Geometry check sheet. Reference: the model listing, model coordinates, mm. A direction names the side the tool comes from. Round coordinates to 2 decimals unless told otherwise and drop trailing zeros. Loops run counter-clockwise (first coordinate to the right, second up) from the corner with the lowest first, then second, coordinate; pieces in that order, holes last.
Autodesk Inventor part; units mm, degrees
ref_plane "YZ Plane" through (0, 0, 0) normal (1, 0, 0) x (0, 1, 0)
ref_plane "XZ Plane" through (0, 0, 0) normal (0, 1, 0) x (-1, 0, 0)
ref_plane "XY Plane" through (0, 0, 0) normal (0, 0, 1) x (1, 0, 0)
sketch "Sketch1" plane through (0, 0, 0) normal (0, 1, 0) x (-1, 0, 0)
  circle A0 centre (0, 0) radius 2.6
  line L0 (0, 0) -> (0, -2.6) construction
  line L1 (0, 0) -> (-2.6, 0) construction
  circle A1 centre (-20, 0) radius 2.6
  circle A2 centre (0, 40) radius 2.6
  circle A3 centre (-20, 40) radius 2.6
  circle A4 centre (0, 80) radius 2.6
  circle A5 centre (-20, 80) radius 2.6
  circle A6 centre (0, -25) radius 2.6
  line L2 (0, -25) -> (2.6, -25) construction
  line L3 (0, -25) -> (0, -27.6) construction
  circle A7 centre (40, -25) radius 2.6
  circle A8 centre (80, -25) radius 2.6
  circle A9 centre (0, -45) radius 2.6
  circle A10 centre (40, -45) radius 2.6
  circle A11 centre (80, -45) radius 2.6
  circle A12 centre (0, 80) radius 5.775 construction
  circle A13 centre (-20, 80) radius 5.775 construction
  circle A14 centre (80, -45) radius 5.775 construction
  circle A15 centre (80, -25) radius 5.775 construction
  line L4 (5.775, 80) -> (5.775, -16.05)
  line L5 (0, 85.775) -> (-20, 85.775)
  arc A16 (5.775, 80) -> (0, 85.775) centre (0, 80) ccw
  arc A17 (-20, 85.775) -> (-25.775, 80) centre (-20, 80) ccw
  line L6 (80, -19.225) -> (8.95, -19.225)
  line L7 (-25.775, 80) -> (-25.775, -47.6)
  line L8 (-22.6, -50.775) -> (80, -50.775)
  arc A18 (-25.775, -47.6) -> (-22.6, -50.775) centre (-22.6, -47.6) ccw
  arc A19 (5.775, -16.05) -> (8.95, -19.225) centre (8.95, -16.05) ccw
  line L9 (85.775, -25) -> (85.775, -45)
  arc A20 (80, -50.775) -> (85.775, -45) centre (80, -45) ccw
  arc A21 (85.775, -25) -> (80, -19.225) centre (80, -25) ccw
  point P0 (-20, -2.6)
  point P1 (-22.6, 0)
  point P2 (0, 37.4)
  point P3 (-2.6, 40)
  point P4 (-20, 37.4)
  point P5 (-22.6, 40)
  point P6 (0, 77.4)
  point P7 (-2.6, 80)
  point P8 (-20, 77.4)
  point P9 (-22.6, 80)
  point P10 (42.6, -25)
  point P11 (40, -27.6)
  point P12 (82.6, -25)
  point P13 (80, -27.6)
  point P14 (2.6, -45)
  point P15 (0, -47.6)
  point P16 (42.6, -45)
  point P17 (40, -47.6)
  point P18 (82.6, -45)
  point P19 (80, -47.6)
  point P20 (5.775, -19.225)
  dimension "d0" = 5.2
  dimension "d3" = 20
  dimension "d6" = 40
  dimension "d13" = 40
  dimension "d16" = 20
  dimension "d19" = 3.175
  dimension "d23" = 25
  dimension "d24" = 3.175
extrude "Extrusion2" add sketch "Sketch1" along normal blind 3
properties part number "CNC-003-StructureGusset3" material "Steel AISI 1080"
1) Mould release check, pull along X, two halves, no side actions. Record for faces 3 (the face through (-45, 1, -19.225)), 4 (the face through (18.6, 1.48, 77.81)), 5 (the face through (-85.775, 1, -35)): +X half, -X half, draft (parallel to the pull), parting line (faces both ways), or undercut.
Report:
face 3: draft
face 4: undercut
face 5: -X half
2) Scan lines: line 1 along Z through (x, y) = (0, 2.3) (3 decimals); line 2 along Z through (x, y) = (-40, 0.7) (3 decimals); line 3 along Z through (x, y) = (20, 0.8) (3 decimals). Record each from-to range of solid material in increasing order.
Report:
line 1: z = -50.775 to -47.6, -42.4 to -27.6, -22.4 to -2.6, 2.6 to 37.4, 42.6 to 77.4, 82.6 to 85.775
line 2: z = -50.775 to -47.6, -42.4 to -27.6, -22.4 to -19.225
line 3: z = -50.775 to -2.6, 2.6 to 37.4, 42.6 to 77.4, 82.6 to 85.775
3) Access from +Z, -Z, +X, -X, +Y, -Y to the whole of each face (thin tool, end or side, straight path). Record for faces 1 (the face through (-5.775, 1, 33)), 2 (the face through (-37.937, 1.479, -43.418)).
Report:
face 1: +Z, -X, +Y, -Y
face 2: +Y, -Y
4) Gauge pin test, flat end, axial feed: pin 1 (0.9 mm diameter, centred on y = 1, z = 55.5, fed in from -X) (3 decimals). Record the tip position at first contact, or that the pin passes through.
Report:
pin 1: stops at x = -5.775
5) Sectioned sample at A-A, the plane z = 0. Record the cut outline in (x, y) (3 decimals).
Report:
outline: (-5.775, 0) - (-2.6, 0) - (-2.6, 3) - (-5.775, 3) - close; (2.6, 0) - (17.4, 0) - (17.4, 3) - (2.6, 3) - close; (22.6, 0) - (25.775, 0) - (25.775, 3) - (22.6, 3) - close
6) Sectioned sample at C-C, the plane z = 34. Record the cut outline in (x, y) (3 decimals), then the cut area to 4 significant figures.
Report:
outline: (-5.775, 0) - (25.775, 0) - (25.775, 3) - (-5.775, 3) - close
area: 94.65 mm2
7) Sectioned sample at B-B, the plane y = 2.5. State how many separate pieces and enclosed holes the cut face has, then the cut area to 3 significant figures.
Report:
separate pieces: 1
enclosed holes: 12
area: 6,550 mm2
